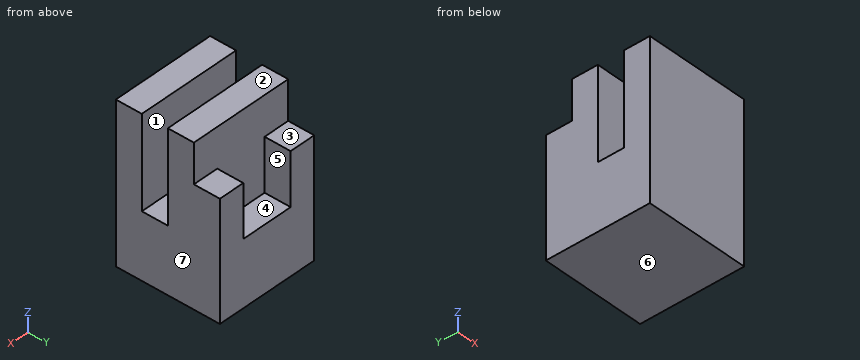
```python
from build123d import *

# Parameters (mm, degrees)
SKETCH1_W           = 40
SKETCH1_H           = 40
BOSS_EXTRUDE1_DEPTH = 60
SKETCH2_W           = 40
SKETCH2_H           = 10
CUT_EXTRUDE1_DEPTH  = 35
SKETCH3_W           = 40
SKETCH3_H           = 10
CUT_EXTRUDE2_DEPTH  = 15
SKETCH4_W           = 20.089198479
SKETCH4_H           = 20.114051596
CUT_EXTRUDE3_DEPTH  = 10


with BuildPart() as part:
    # Sketch1 → Boss-Extrude1 (new body)
    with BuildSketch(Plane.XY):
        with Locations((20, 20)):
            Rectangle(SKETCH1_W, SKETCH1_H)
    extrude(amount=BOSS_EXTRUDE1_DEPTH)

    # Sketch2 → Cut-Extrude1 (cut)
    with BuildSketch(Plane.XY.offset(60)):
        with Locations((20, 15)):
            Rectangle(SKETCH2_W, SKETCH2_H)
    extrude(amount=-CUT_EXTRUDE1_DEPTH, mode=Mode.SUBTRACT)

    # Sketch3 → Cut-Extrude2 (cut)
    with BuildSketch(Plane.XY.offset(60)):
        with Locations((20, 35)):
            Rectangle(SKETCH3_W, SKETCH3_H)
    extrude(amount=-CUT_EXTRUDE2_DEPTH, mode=Mode.SUBTRACT)

    # Sketch4 → Cut-Extrude3 (cut)
    with BuildSketch(Plane(origin=(0, 40, 0), x_dir=(1, 0, 0), z_dir=(0, 1, 0))):
        with Locations((20.04459924, -34.942974202)):
            Rectangle(SKETCH4_W, SKETCH4_H)
    extrude(amount=-CUT_EXTRUDE3_DEPTH, mode=Mode.SUBTRACT)


solid = part.part
```
Design review of the part built by this model. Coordinates are the model's own, in mm. Face numbers are marked on the shaded views. A direction names the side the tool comes from. Coordinates: 2 decimals unless noted, no trailing zeros. Write each loop counter-clockwise with the first axis right and the second up, starting at its lowest first coordinate (ties: lowest second). Pieces come first, ordered by that corner, then holes.
1) Insertion check: pin 1 (3 mm diameter, centred on x = 6, y = 36, fed in from +Z); pin 2 (3 mm diameter, centred on x = 20, y = 33.5, fed in from +Z); pin 3 (5 mm diameter, centred on x = 9, z = 53, fed in from +Y). Each pin has a flat end and moves straight along its axis. Give the tip position at first contact, or say it passes through.
2) Machinability: for the marked faces 1, 2, 3 and 4, which of the approach directions +Z, -Z, +X, -X, +Y, -Y give a long, thin tool a straight path to every point of the face, cutting with its end or side? Answer none if there is none.
3) Add section B-B (x = 3). Write out the cut boundary in (y, z).
4) Add section D-D (y = 12). Write out the cut boundary in (x, z).
5) Add section A-A (z = 48). Write out the cut boundary in (x, y).
6) Mouldability with a two-part tool opening along X and no side actions: class the marked faces 5, 6 and 7 as +X half, -X half, draft (parallel to the pull), parting line (faces both ways), or undercut.
7) To check wall thickness, follow L1, parallel to Y at x = 22, z = 51.5; L2, parallel to Y at x = 36, z = 42; L3, parallel to Z at x = 4, y = 16. State the ranges of each line that lie inside material, in increasing order.
8) Add section C-C (z = 33). Write out the cut boundary in (x, y).
Check result:
1. pin 1: stops at z = 45
1. pin 2: stops at z = 24.89
1. pin 3: stops at y = 30
2. face 1: +Z, +X, -X
2. face 2: +Z, +X, -X, +Y, -Y
2. face 3: +Z, +X, -X, +Y
2. face 4: +Z, +Y
3. outline: (0, 0) - (40, 0) - (40, 45) - (30, 45) - (30, 60) - (20, 60) - (20, 25) - (10, 25) - (10, 60) - (0, 60) - close
4. outline: (0, 0) - (40, 0) - (40, 25) - (0, 25) - close
5. outline: (0, 0) - (40, 0) - (40, 10) - (0, 10) - close; (0, 20) - (40, 20) - (40, 30) - (0, 30) - close
6. face 5: undercut
6. face 6: draft
6. face 7: +X half
7. L1: y = 0 to 10, 20 to 30
7. L2: y = 0 to 10, 20 to 40
7. L3: z = 0 to 25
8. outline: (0, 0) - (40, 0) - (40, 10) - (0, 10) - close; (0, 20) - (40, 20) - (40, 40) - (30.09, 40) - (30.09, 30) - (10, 30) - (10, 40) - (0, 40) - close
